```python
from build123d import *

# Parameters (mm, degrees)
F0_R     = 11.65
F1_DEPTH = 2.2
F3_DEPTH = 25


with BuildPart() as f1:
    # F0 (on Top) → F1 (new body)
    with BuildSketch(Plane.XY):
        Circle(F0_R)
    extrude(amount=F1_DEPTH)

    # F2 (on face) → F3 (cut)
    with BuildSketch(Plane(origin=(0, 0, 0), x_dir=(1, 0, 0), z_dir=(0, 0, -1))):
        with BuildLine():
            ThreePointArc((-6.1164736573, -6.1164736573), (-3.31021169, -7.9915579562), (0, -8.65))
            Line((0, -8.65), (0, -6.65))
            ThreePointArc((0, -6.65), (-2.5448448252, -6.1437988912), (-4.7022600949, -4.7022600949))
            Line((-4.7022600949, -4.7022600949), (-6.1164736573, -6.1164736573))
        make_face()
        with BuildLine():
            ThreePointArc((-3.2880465325, -3.2880465325), (-1.7794779605, -4.2960398262), (0, -4.65))
            Line((0, -4.65), (0, -2.65))
            ThreePointArc((0, -2.65), (-1.0141110958, -2.4482807612), (-1.8738329701, -1.8738329701))
            Line((-1.8738329701, -1.8738329701), (-3.2880465325, -3.2880465325))
        make_face()
        with BuildLine():
            ThreePointArc((6.1164736573, -6.1164736573), (7.9915579562, -3.31021169), (8.65, 0))
            Line((8.65, 0), (6.65, 0))
            ThreePointArc((6.65, 0), (6.1437988912, -2.5448448252), (4.7022600949, -4.7022600949))
            Line((4.7022600949, -4.7022600949), (6.1164736573, -6.1164736573))
        make_face()
        with BuildLine():
            ThreePointArc((3.2880465325, -3.2880465325), (4.2960398262, -1.7794779605), (4.65, 0))
            Line((4.65, 0), (2.65, 0))
            ThreePointArc((2.65, 0), (2.4482807612, -1.0141110958), (1.8738329701, -1.8738329701))
            Line((1.8738329701, -1.8738329701), (3.2880465325, -3.2880465325))
        make_face()
        with BuildLine():
            Line((4.7022600949, 4.7022600949), (6.1164736573, 6.1164736573))
            ThreePointArc((6.1164736573, 6.1164736573), (3.31021169, 7.9915579562), (0, 8.65))
            Line((0, 8.65), (0, 6.65))
            ThreePointArc((0, 6.65), (2.5448448252, 6.1437988912), (4.7022600949, 4.7022600949))
        make_face()
        with BuildLine():
            Line((1.8738329701, 1.8738329701), (3.2880465325, 3.2880465325))
            ThreePointArc((3.2880465325, 3.2880465325), (1.7794779605, 4.2960398262), (0, 4.65))
            Line((0, 4.65), (0, 2.65))
            ThreePointArc((0, 2.65), (1.0141110958, 2.4482807612), (1.8738329701, 1.8738329701))
        make_face()
        with BuildLine():
            Line((-1.8738329701, 1.8738329701), (-3.2880465325, 3.2880465325))
            ThreePointArc((-3.2880465325, 3.2880465325), (-4.2960398262, 1.7794779605), (-4.65, 0))
            Line((-4.65, 0), (-2.65, 0))
            ThreePointArc((-2.65, 0), (-2.4482807612, 1.0141110958), (-1.8738329701, 1.8738329701))
        make_face()
        with BuildLine():
            Line((-4.7022600949, 4.7022600949), (-6.1164736573, 6.1164736573))
            ThreePointArc((-6.1164736573, 6.1164736573), (-7.9915579562, 3.31021169), (-8.65, 0))
            Line((-8.65, 0), (-6.65, 0))
            ThreePointArc((-6.65, 0), (-6.1437988912, 2.5448448252), (-4.7022600949, 4.7022600949))
        make_face()
    extrude(amount=-F3_DEPTH, mode=Mode.SUBTRACT)


solid = f1.part
```
Build history of the part. All positions in model axes, mm. A direction names the side the tool comes from. Coordinates: 2 decimals unless noted, no trailing zeros. Order: outer loops, then holes, each group sorted by start corner. A loop starts at its lowest first (then second) coordinate and runs counter-clockwise, first axis right, second up. Notation, with made-up numbers: (-31, 54) -> (1, 54) arc R25 ccw to (1, 92) -> close; hole circle Ø6 at (-28, 68). An arc over 180 degrees is marked (long way). Answer in a Markdown table with one row per item. Add a question column.
Q1. Drop flat-ended pins along their axis: pin 1 (1 mm diameter, centred on x = 4.5, z = 0.5, fed in from -Y); pin 2 (0.6 mm diameter, centred on y = -4, z = 0.5, fed in from +X); pin 3 (1 mm diameter, centred on x = 8, z = 1.5, fed in from +Y); pin 4 (8 mm diameter, centred on x = 9.5, y = 0, fed in from -Z). Give the stop position or say it passes through.
Q2. Which spindle directions (+Z, -Z, +X, -X, +Y, -Y) get a long thin tool onto all of the face, cutting with end or side? Do faces 1 (the face through (-5, 5, 1)), 2 (the face through (0, 0, 2.2)). Say none if no direction does.
Q3. Band-saw the part on D-D, the plane y = 4.25. List the corners of the cut face in (x, z), then the cut area to 3 significant figures.
Q4. Band-saw the part on A-A, the plane z = 1.7. Give the number of separate pieces and of enclosed holes in the cut face, then the cut area to 3 significant figures.
Q5. Wall check: line 1 along X through (y, z) = (0.75, 1); line 2 along Y through (x, z) = (6, 2.05); line 3 along Y through (x, z) = (5, 2.1). Give the ranges that are in metal, low to high. Write a range as [from, to].
Q6. Mould opens along Y. For faces 3 (the face through (-2.53, -11.37, 1.08)), 4 (the face through (-1.001, 2.454, 1.085)), 5 (the face through (0, 0, 0)) say: +Y half, -Y half, draft (parallel to the pull), parting line (faces both ways), or undercut.
Q7. Band-saw the part on C-C, the plane x = -4. List the corners of the cut face in (y, z).
Q8. Band-saw the part on B-B, the plane x = -7. List the corners of the cut face in (y, z).
Answers follow:
| question | item | result |
|---|---|---|
| 1 | pin 1 | y = -10.94 |
| 1 | pin 2 | x = 11.05 |
| 1 | pin 3 | y = 8.91 |
| 1 | pin 4 | z = 0 |
| 2 | face 1 | +Z, -Z |
| 2 | face 2 | +Z, +X, -X, +Y, -Y |
| 3 | outline | (-10.85, 0) -> (-1.89, 0) -> (-1.89, 2.2) -> (-10.85, 2.2) -> close; (0, 0) -> (5.11, 0) -> (5.11, 2.2) -> (0, 2.2) -> close; (7.53, 0) -> (10.85, 0) -> (10.85, 2.2) -> (7.53, 2.2) -> close |
| 3 | area | 38.3 mm^2 |
| 4 | separate pieces | 1 |
| 4 | enclosed holes | 8 |
| 4 | area | 355 mm^2 |
| 5 | line 1 | [-11.63, 2.54], [4.59, 6.61], [8.62, 11.63] |
| 5 | line 2 | [-9.99, -6.23], [-6, 2.87], [6, 9.99] |
| 5 | line 3 | [-10.52, -7.06], [-5, 4.38], [5, 10.52] |
| 6 | face 3 | parting line |
| 6 | face 4 | undercut |
| 6 | face 5 | draft |
| 7 | outline | (-10.94, 0) -> (-2.37, 0) -> (-2.37, 2.2) -> (-10.94, 2.2) -> close; (0, 0) -> (5.31, 0) -> (5.31, 2.2) -> (0, 2.2) -> close; (7.67, 0) -> (10.94, 0) -> (10.94, 2.2) -> (7.67, 2.2) -> close |
| 8 | outline | (-9.31, 0) -> (-5.08, 0) -> (-5.08, 2.2) -> (-9.31, 2.2) -> close; (0, 0) -> (9.31, 0) -> (9.31, 2.2) -> (0, 2.2) -> close |
